Geometry: see drawing. Coordinates: mm, zero at the bounding-box minimum. A direction names the side the tool comes from. Give positions to 0.01 mm unless a question says otherwise; leave off trailing zeros. Order: outer loops, then holes, each group sorted by start corner. A loop starts at its lowest first (then second) coordinate and runs counter-clockwise, first axis right, second up. Notation, with made-up numbers: (21, -8.5) - (70, -8.5) arc R20 ccw to (70, -1.5) - close; hole circle Ø8 at (28.25, -16.5). An arc over 180 degrees is marked (long way). One line per item, written item: value. Start each with the question number.
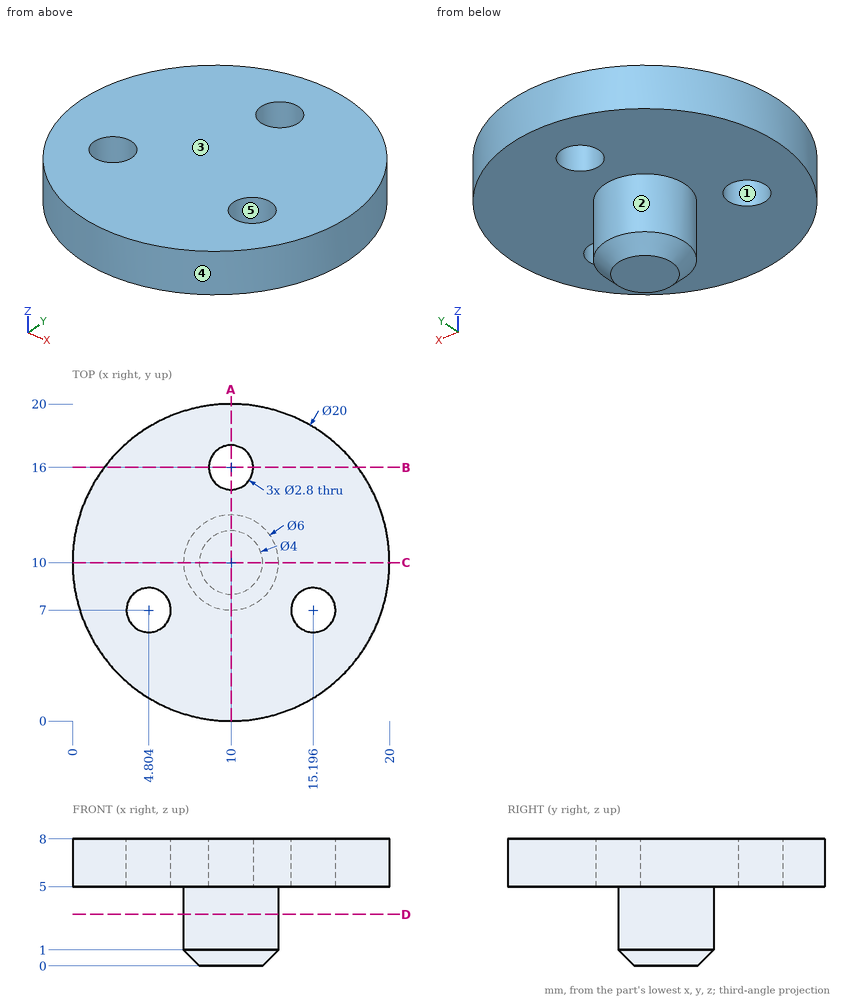
1. Section A-A on x = 10. Return the cut outline in (y, z), then the cut area to 3 significant figures.
2. Section D-D on z = 3.25. Return the cut outline in (x, y).
3. Set-up query: the marked faces 1 and 2. Return all of +Z, -Z, +X, -X, +Y, -Y with unobstructed straight access to the full face (end or side cutting, diameter ignored); none if empty.
4. Section B-B on y = 16. Return the cut outline in (x, z), then the cut area to 3 significant figures.
5. Section C-C on y = 10. Return the cut outline in (x, z).
6. Ray query, L1, parallel to Y at x = 10, z = 5.75; L2, parallel to X at y = 7, z = 6.3; L3, parallel to Z at x = 7.25, y = 3.5. Return the intervals inside material, ascending.
7. Draft query along Y for the marked faces 3, 4 and 5. Return one class per face: pulls with the +Y half, pulls with the -Y half, needs draft (parallel to the pull), parting line crosses it, or undercut.
8. Contact query for flat-ended pins moving along their axis: pin 1 Ø1.5 at (x, z) = (12, 4.5) entering from -Y; pin 2 Ø3 at (x, z) = (12.5, 6) entering from +Y. Output: stop coordinate, or through.
Data:
1. outline: (0, 5) - (7, 5) - (7, 1) - (8, 0) - (12, 0) - (13, 1) - (13, 5) - (14.6, 5) - (14.6, 8) - (0, 8) - close; (17.4, 5) - (20, 5) - (20, 8) - (17.4, 8) - close
1. area: 80.6 mm2
2. outline: circle Ø6 at (10, 10)
3. face 1: +Z, -Z
3. face 2: -Z
4. outline: (2, 5) - (8.6, 5) - (8.6, 8) - (2, 8) - close; (11.4, 5) - (18, 5) - (18, 8) - (11.4, 8) - close
4. area: 39.6 mm2
5. outline: (0, 5) - (7, 5) - (7, 1) - (8, 0) - (12, 0) - (13, 1) - (13, 5) - (20, 5) - (20, 8) - (0, 8) - close
6. L1: y = 0 to 14.6, 17.4 to 20
6. L2: x = 0.46 to 3.4, 6.2 to 13.8, 16.6 to 19.54
6. L3: z = 5 to 8
7. face 3: needs draft
7. face 4: parting line crosses it
7. face 5: undercut
8. pin 1: stops at y = 0.1
8. pin 2: stops at y = 19.95
